from build123d import *

# Parameters (mm, degrees)
F1_DEPTH = 20
F0_W     = 30
F0_H     = 30
F2_DEPTH = 10
F3_R     = 3


with BuildPart() as f1:
    # F0 (on Top) → F1 (new body)
    with BuildSketch(Plane.XY):
        Polygon((-20, -20), (20, -20), (20, -10), (-10, -10), (-10, 20), (-20, 20), align=None)
    extrude(amount=F1_DEPTH)

    # F0 (on Top) → F2 (join)
    with BuildSketch(Plane.XY):
        with Locations((5, 5)):
            Rectangle(F0_W, F0_H)
    extrude(amount=F2_DEPTH)

    # F3
    f3_edges = [f1.edges().sort_by_distance(p)[0] for p in [
        (-10, -10, 15),
    ]]
    fillet(f3_edges, radius=F3_R)


solid = f1.part
Could you check a few things on this model? Use its own coordinates, in mm. A direction names the side the tool comes from. Coordinates: 2 decimals unless noted, no trailing zeros. Write each loop counter-clockwise with the first axis right and the second up, starting at its lowest first coordinate (ties: lowest second). Pieces come first, ordered by that corner, then holes. Notation, with made-up numbers: M 33.25,29 L 40.25,29 A18 ccw 40.25,38 Z; hole C 83.25,58.5 d7. An arc over 180 degrees is marked long. One line per question, with ' | ' between items.
1) For pin 1 Ø3 at (y, z) = (0, 13.5) entering from +X; pin 2 Ø8 at (x, y) = (5, 4) entering from +Z; pin 3 Ø2 at (x, z) = (7, 17.5) entering from +Y, each with a flat end and sliding along its axis, tell me the tip position at first contact or that it passes through.
Checks:
pin 1: x = -10 | pin 2: z = 10 | pin 3: y = -10
2) Imagine slicing it at A-A, the plane z = 12.75. Write out the boundary of the cut face in (x, y), and give its area (3 significant figures).
Checks:
outline: M -20,-20 L 20,-20 L 20,-10 L -7,-10 A3 cw -10,-7 L -10,20 L -20,20 Z | area: 702 mm²
3) I need wall thicknesses on probe 1 along Z at (x, y) = (4.5, 7); probe 2 along X at (y, z) = (17, 13.5). Which ranges of each line are inside material? Lowest first, please. Write a range as [from, to].
Checks:
probe 1: [0, 10] | probe 2: [-20, -10]
4) For faces 1 (the face through (0, -20, 10)), 2 (the face through (-10, 6, 15)), which set-ups out of +Z, -Z, +X, -X, +Y, -Y let a thin tool reach every point of the face, with its end or its side?
Checks:
face 1: +Z, -Z, +X, -X, -Y | face 2: +Z, +X, +Y
5) Imagine slicing it at B-B, the plane x = 15.5. Write out the boundary of the cut face in (y, z), and give its area (3 significant figures).
Checks:
outline: M -20,0 L 20,0 L 20,10 L -10,10 L -10,20 L -20,20 Z | area: 500 mm²
